The model under review builds one solid part; all positions refer to its coordinate system, in mm. A direction names the side the tool comes from. Coordinates: 2 decimals unless noted, no trailing zeros. Write each loop counter-clockwise with the first axis right and the second up, starting at its lowest first coordinate (ties: lowest second). Pieces come first, ordered by that corner, then holes. Notation, with made-up numbers: (56, -18.5) - (94, -18.5) arc R31 ccw to (94, 7.5) - close; hole circle Ø11 at (21, -39.75). An arc over 180 degrees is marked (long way). Put each result on its own line as item: value. Start each with the question number.
Item 1: To check wall thickness, follow L1, parallel to X at y = 0, z = 42; L2, parallel to X at y = 0, z = 28.5. State the ranges of each line that lie inside material, in increasing order. Write a range as [from, to].
Item 2: For pin 1 (8.5 mm diameter, centred on x = 0, y = 0, fed in from -Z); pin 2 (8.5 mm diameter, centred on x = 27.5, y = 7, fed in from +Z); pin 3 (14.5 mm diameter, centred on x = 26.5, y = 5.5, fed in from -Z); pin 4 (2 mm diameter, centred on y = -9, z = 34, fed in from -X), all flat-tipped, find the tip position at first contact; note any pin that passes through.
Item 3: Consider section B-B on z = 25.5. Give the boundary of the cut face in (x, y) (1 decimal).
Item 4: Mouldability with a two-part tool opening along X and no side actions: class faces 4 (the face through (0, 6, 50.8)), 5 (the face through (-13.63, -4.29, 41.14)), 6 (the face through (0, 5, 38.1)) as pulls with the +X half, pulls with the -X half, needs draft (parallel to the pull), parting line crosses it, or undercut.
Item 5: Consider section D-D on x = -10. Give the boundary of the cut face in (y, z).
Item 6: Machinability: for faces 1 (the face through (-13.63, -4.29, 9.39)), 2 (the face through (38.1, 0, 25)), 3 (the face through (0, 5, 44.45)), which of the approach directions +Z, -Z, +X, -X, +Y, -Y give a long, thin tool a straight path to every point of the face, cutting with its end or side? Answer none if there is none.
Item 7: Consider section A-A on y = 0. Give the boundary of the cut face in (x, z), then the cut area to 3 significant figures.
Item 8: Consider section C-C on y = -5.75. Give the boundary of the cut face in (x, z).
```python
from build123d import *

# Parameters (mm, degrees)
F4_DEPTH = 12.7
F5_R     = 4.7625
F6_DEPTH = 50.801


with BuildPart() as f1:
    # F0 (on Front) → F1 (revolve)
    with BuildSketch(Plane.XZ):
        Polygon((-4.7625, 44.45), (-4.7625, 50.8), (-14.2875, 50.8), (-14.2875, 0), (-4.7625, 0), (-4.7625, 38.1), (-7.9375, 38.1), (-7.9375, 44.45), align=None)
    revolve(axis=Axis((0, 0, 5.547127), (0, 0, 1)))

    # F3 (on offset) → F4 (join)
    with BuildSketch(Plane.XY.offset(19.05)):
        with BuildLine():
            Line((0, 14.2875), (-38.1, 14.2875))
            Line((-38.1, 14.2875), (-38.1, -14.2875))
            Line((-38.1, -14.2875), (0, -14.2875))
            ThreePointArc((0, -14.2875), (-14.2875, 0), (0, 14.2875))
        make_face()
        with BuildLine():
            Line((38.1, 14.2875), (0, 14.2875))
            ThreePointArc((0, 14.2875), (10.102788, 10.102788), (14.2875, 0))
            ThreePointArc((14.2875, 0), (10.102788, -10.102788), (0, -14.2875))
            Line((0, -14.2875), (38.1, -14.2875))
            Line((38.1, -14.2875), (38.1, 14.2875))
        make_face()
    extrude(amount=F4_DEPTH)

    # F5 (on face) → F6 (cut, through all)
    with BuildSketch(Plane.XY.offset(50.8)):
        Circle(F5_R)
    extrude(amount=-F6_DEPTH, mode=Mode.SUBTRACT)


solid = f1.part
```
Report:
1. L1: [-14.29, -7.94], [7.94, 14.29]
1. L2: [-38.1, -4.76], [4.76, 38.1]
2. pin 1: through
2. pin 2: z = 31.75
2. pin 3: z = 19.05
2. pin 4: x = -11.84
3. outline: (-38.1, -14.3) - (38.1, -14.3) - (38.1, 14.3) - (-38.1, 14.3) - close; hole circle Ø9.5 at (0, 0)
4. face 4: needs draft
4. face 5: parting line crosses it
4. face 6: undercut
5. outline: (-14.29, 19.05) - (-10.2, 19.05) - (-10.2, 0) - (10.2, 0) - (10.2, 19.05) - (14.29, 19.05) - (14.29, 31.75) - (10.2, 31.75) - (10.2, 50.8) - (-10.2, 50.8) - (-10.2, 31.75) - (-14.29, 31.75) - close
6. face 1: -Z
6. face 2: +Z, -Z, +X, +Y, -Y
6. face 3: none
7. outline: (-38.1, 19.05) - (-14.29, 19.05) - (-14.29, 0) - (-4.76, 0) - (-4.76, 38.1) - (-7.94, 38.1) - (-7.94, 44.45) - (-4.76, 44.45) - (-4.76, 50.8) - (-14.29, 50.8) - (-14.29, 31.75) - (-38.1, 31.75) - close; (4.76, 0) - (14.29, 0) - (14.29, 19.05) - (38.1, 19.05) - (38.1, 31.75) - (14.29, 31.75) - (14.29, 50.8) - (4.76, 50.8) - (4.76, 44.45) - (7.94, 44.45) - (7.94, 38.1) - (4.76, 38.1) - close
7. area: 1,530 mm²
8. outline: (-38.1, 19.05) - (-13.08, 19.05) - (-13.08, 0) - (13.08, 0) - (13.08, 19.05) - (38.1, 19.05) - (38.1, 31.75) - (13.08, 31.75) - (13.08, 50.8) - (-13.08, 50.8) - (-13.08, 31.75) - (-38.1, 31.75) - close; hole (-5.47, 38.1) - (5.47, 38.1) - (5.47, 44.45) - (-5.47, 44.45) - close
